For this review, use the dimensioned drawing (mm, ordinates from the lowest corner) and the shaded views. A direction names the side the tool comes from. Coordinates: 2 decimals unless noted, no trailing zeros. Order: outer loops, then holes, each group sorted by start corner. A loop starts at its lowest first (then second) coordinate and runs counter-clockwise, first axis right, second up. Notation, with made-up numbers: M 89.25,18 L 130.25,18 A15 cw 130.25,35 Z; hole C -2.75,-35 d10. An arc over 180 degrees is marked long. Write each question's results on one line, items separated by ' | '.
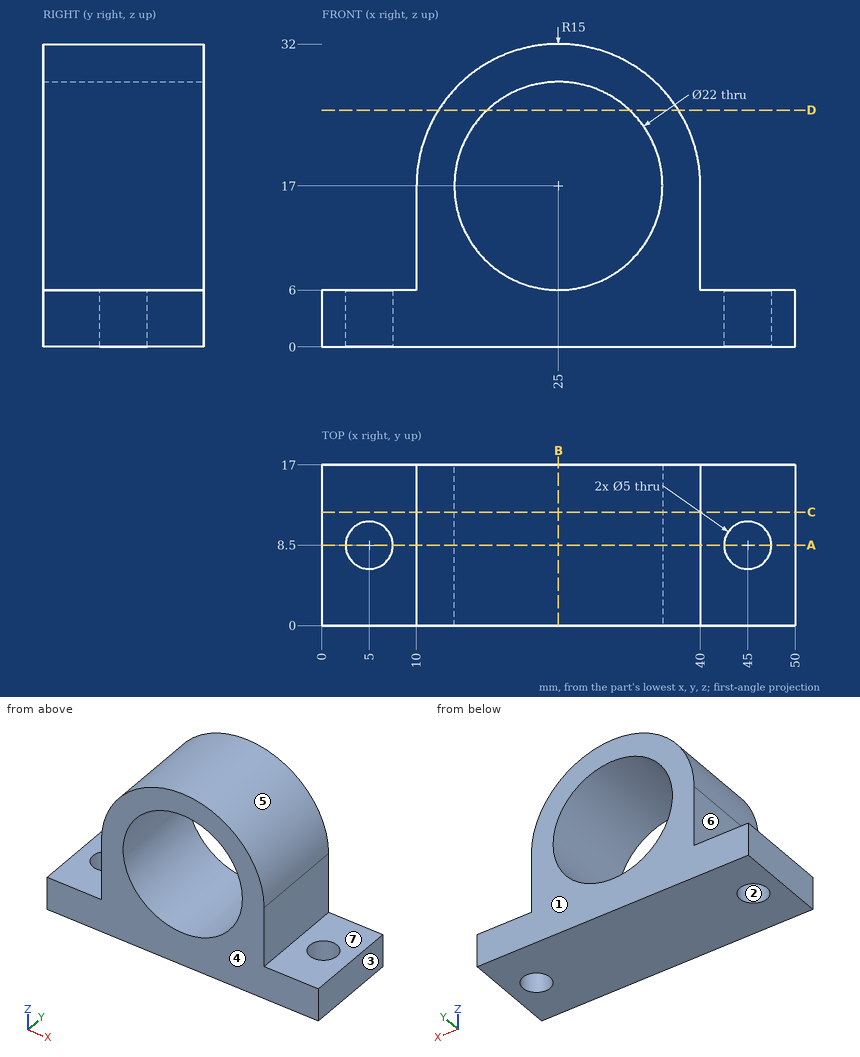
1) Take a section at A-A on y = 8.5. State the section outline as (x, z) points.
Solutions:
outline: M 0,0 L 2.5,0 L 2.5,6 L 0,6 Z; M 7.5,0 L 42.5,0 L 42.5,6 L 40,6 L 40,17 A15 ccw 10,17 L 10,6 L 7.5,6 Z; M 47.5,0 L 50,0 L 50,6 L 47.5,6 Z; hole C 25,17 d22
2) Take a section at D-D on z = 25. State the section outline as (x, y) points.
Solutions:
outline: M 12.31,0 L 17.45,0 L 17.45,17 L 12.31,17 Z; M 32.55,0 L 37.69,0 L 37.69,17 L 32.55,17 Z
3) To check wall thickness, follow line 1 along Y through (x, z) = (5, 3.7); line 2 along Z through (x, y) = (25, 8); line 3 along X through (y, z) = (7.75, 23). State the ranges of each line that lie inside material, in increasing order.
Solutions:
line 1: 0 to 6, 11 to 17 | line 2: 0 to 6, 28 to 32 | line 3: 11.25 to 15.78, 34.22 to 38.75
4) Take a section at C-C on y = 12. State the section outline as (x, z) points, plus the area to 3 significant figures.
Solutions:
outline: M 0,0 L 50,0 L 50,6 L 40,6 L 40,17 A15 ccw 10,17 L 10,6 L 0,6 Z; hole C 25,17 d22 | area: 603 mm2
5) The part is to be moulded in two halves that separate along Y. For the marked faces 1, 2, 3 and 4, say which applies: pulls with the +Y half, pulls with the -Y half, needs draft (parallel to the pull), parting line crosses it, or undercut.
Solutions:
face 1: pulls with the +Y half | face 2: undercut | face 3: needs draft | face 4: pulls with the -Y half
6) Take a section at B-B on x = 25. State the section outline as (y, z) points, plus the area to 3 significant figures.
Solutions:
outline: M 0,0 L 17,0 L 17,6 L 0,6 Z; M 0,28 L 17,28 L 17,32 L 0,32 Z | area: 170 mm2
7) For pin 1 (6.5 mm diameter, centred on x = 45, y = 8.5, fed in from +Z); pin 2 (4 mm diameter, centred on y = 11.5, z = 21, fed in from +X); pin 3 (4 mm diameter, centred on y = 8, z = 15.5, fed in from +X); pin 4 (4.5 mm diameter, centred on x = 5, y = 8.5, fed in from +Z), all flat-tipped, find the tip position at first contact; note any pin that passes through.
Solutions:
pin 1: z = 6 | pin 2: x = 39.87 | pin 3: x = 40 | pin 4: through
8) For the marked faces 5, 6 and 7, list the 3-axis set-ups (+Z, -Z, +X, -X, +Y, -Y) from which the entire face can be reached by the end or side of a thin tool; tool diameter is ignored.
Solutions:
face 5: +Z, +Y, -Y | face 6: +Z, -X, +Y, -Y | face 7: +Z, +X, +Y, -Y
